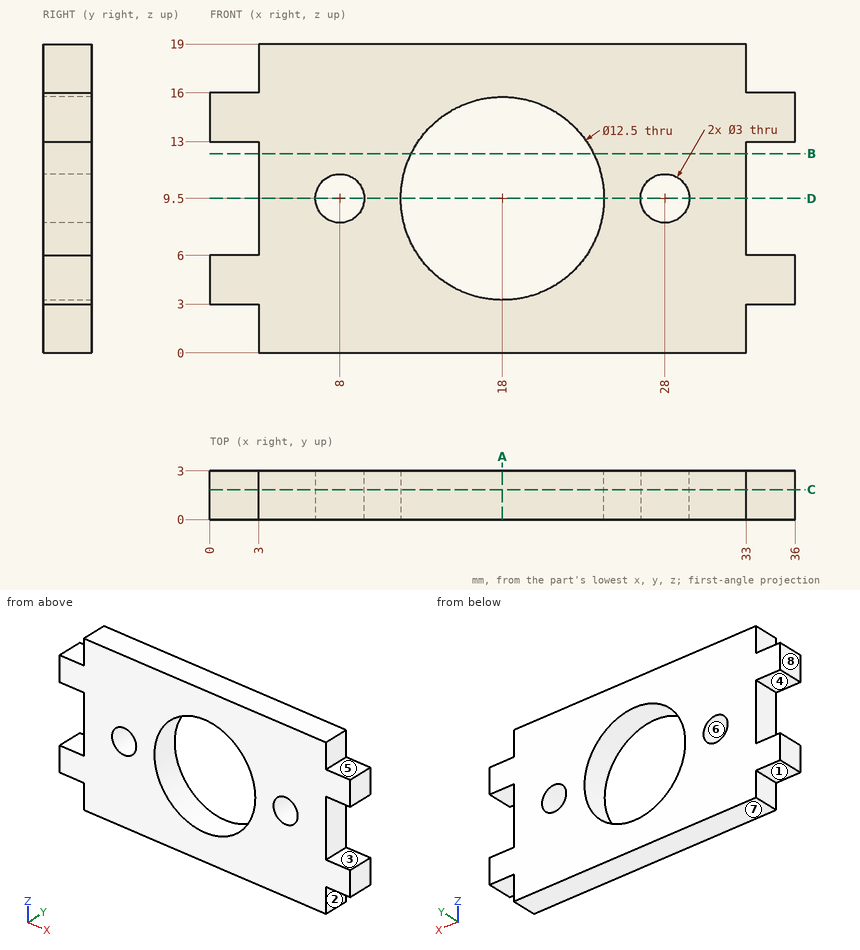
The figure shows three views and two pictorial views of one solid part (mm, origin at its lowest corner). Answer the questions. A direction names the side the tool comes from. Give positions to 0.01 mm unless a question says otherwise; leave off trailing zeros. Write each loop counter-clockwise with the first axis right and the second up, starting at its lowest first coordinate (ties: lowest second). Pieces come first, ordered by that corner, then holes. Notation, with made-up numbers: (50, 31.5) - (71, 31.5) arc R21 ccw to (71, 63.5) - close; hole circle Ø3 at (33.5, 55). An arc over 180 degrees is marked (long way). Return JSON: item names as keys, results as strings.
Q1. Given P1, Ø0.9, axis at y = 1.5, z = 18, coming from the -X side; P2, Ø1, axis at x = 4.5, y = 0.5, coming from the -Z side; P3, Ø1.5, axis at x = 1.5, y = 1, coming from the -Z side; P4, Ø1.5, axis at y = 1, z = 17, coming from the +X side, each flat-ended and moving along its own axis, determine where each tip first touches the part or whether it passes through.
Reply:
{"P1": "x = 3", "P2": "z = 0", "P3": "z = 3", "P4": "x = 33"}
Q2. For the marked faces 1, 2, 3, 4 and 5, determine the directions among +Z, -Z, +X, -X, +Y, -Y from which every point of the face is accessible in a straight line to the end or side of a thin tool.
Reply:
{"face 1": "-Z, -X, +Y, -Y", "face 2": "-Z, +X, +Y, -Y", "face 3": "+X, +Y, -Y", "face 4": "-X, +Y, -Y", "face 5": "+Z, +X, +Y, -Y"}
Q3. Consider line 1 along X through (y, z) = (1.7, 9.5); line 2 along Z through (x, y) = (28, 1.55); line 3 along Z through (x, y) = (34, 2.75). Determine where each line is inside the solid, lowest interval first. Write a range as [from, to].
Reply:
{"line 1": "[3, 6.5], [9.5, 11.75], [24.25, 26.5], [29.5, 33]", "line 2": "[0, 8], [11, 19]", "line 3": "[3, 6], [13, 16]"}
Q4. A cutting plane is placed at B-B, the plane z = 12.25. Determine the outline of the cut face in (x, y), and give its area (3 significant figures).
Reply:
{"outline": "(3, 0) - (12.39, 0) - (12.39, 3) - (3, 3) - close; (23.61, 0) - (33, 0) - (33, 3) - (23.61, 3) - close", "area": "56.3 mm²"}
Q5. A cutting plane is placed at D-D, the plane z = 9.5. Determine the outline of the cut face in (x, y), and give its area (3 significant figures).
Reply:
{"outline": "(3, 0) - (6.5, 0) - (6.5, 3) - (3, 3) - close; (9.5, 0) - (11.75, 0) - (11.75, 3) - (9.5, 3) - close; (24.25, 0) - (26.5, 0) - (26.5, 3) - (24.25, 3) - close; (29.5, 0) - (33, 0) - (33, 3) - (29.5, 3) - close", "area": "34.5 mm²"}
Q6. A cutting plane is placed at C-C, the plane y = 1.85. Determine the outline of the cut face in (x, z).
Reply:
{"outline": "(0, 3) - (3, 3) - (3, 0) - (33, 0) - (33, 3) - (36, 3) - (36, 6) - (33, 6) - (33, 13) - (36, 13) - (36, 16) - (33, 16) - (33, 19) - (3, 19) - (3, 16) - (0, 16) - (0, 13) - (3, 13) - (3, 6) - (0, 6) - close; hole circle Ø3 at (8, 9.5); hole circle Ø12.5 at (18, 9.5); hole circle Ø3 at (28, 9.5)"}
Q7. For a pull along X with two mould halves and no side action, classify the marked faces 6, 7 and 8 as released by +X, released by -X, zero draft, split by the parting line, or undercut.
Reply:
{"face 6": "undercut", "face 7": "zero draft", "face 8": "released by -X"}
Q8. A cutting plane is placed at A-A, the plane x = 18. Determine the outline of the cut face in (y, z).
Reply:
{"outline": "(0, 0) - (3, 0) - (3, 3.25) - (0, 3.25) - close; (0, 15.75) - (3, 15.75) - (3, 19) - (0, 19) - close"}
